from build123d import *

# Parameters (mm, degrees)
SKETCH_1_R      = 1
SKETCH_1_R_2    = 2
EXTRUDE_1_DEPTH = 2


with BuildPart() as part:
    # Эскиз1 → Бобышка-Вытянуть1 (new body)
    with BuildSketch(Plane(origin=(0, 0, 0), x_dir=(1, 0, 0), z_dir=(0, 1, 0))):
        with BuildLine():
            Line((8, 25.5), (48.3, 25.5))
            Line((48.3, 25.5), (48.3, 16))
            Line((48.3, 16), (56.3, 16))
            Line((56.3, 16), (56.3, 14))
            Line((56.3, 14), (48.3, 14))
            Line((48.3, 14), (48.3, 4.5))
            Line((48.3, 4.5), (8, 4.5))
            Line((8, 4.5), (8, 14))
            Line((8, 14), (0, 14))
            Line((0, 14), (0, 0))
            Line((0, 0), (75.8, 0))
            ThreePointArc((75.8, 0), (90.8, 15), (75.8, 30))
            Line((75.8, 30), (0, 30))
            Line((0, 30), (0, 16))
            Line((0, 16), (8, 16))
            Line((8, 16), (8, 25.5))
        make_face()
        with Locations(Location((3.4, 10, 0), (0, 0, 270))):
            Circle(SKETCH_1_R, mode=Mode.SUBTRACT)
        with Locations(Location((3.4, 20, 0), (0, 0, 270))):
            Circle(SKETCH_1_R, mode=Mode.SUBTRACT)
        with Locations(Location((52.6, 10, 0), (0, 0, 270))):
            Circle(SKETCH_1_R, mode=Mode.SUBTRACT)
        with Locations(Location((52.6, 20, 0), (0, 0, 270))):
            Circle(SKETCH_1_R, mode=Mode.SUBTRACT)
        with Locations(Location((75.8, 15, 0), (0, 0, 270))):
            Circle(SKETCH_1_R_2, mode=Mode.SUBTRACT)
    extrude(amount=EXTRUDE_1_DEPTH)


solid = part.part
CAD build for the part. Positions are in the model's coordinates, mm. A direction names the side the tool comes from. Round coordinates to 2 decimals unless told otherwise and drop trailing zeros. Loops run counter-clockwise (first coordinate to the right, second up) from the corner with the lowest first, then second, coordinate; pieces in that order, holes last. Notation, with made-up numbers: M -18,26.25 L 19,26.25 A29 ccw 19,55.25 Z; hole C 28.5,-18 d7. An arc over 180 degrees is marked long. One line per question, with ' | ' between items. Start each with the question number.
Item 1: Cut at A-A, the plane x = 39.5. Write the cut outline in (y, z).
Item 2: Cut at B-B, the plane y = 0.5. Write the cut outline in (x, z), plus the area to 3 significant figures.
Item 3: Wall check: line 1 (Z direction, x = 22, y = 0.35); line 2 (X direction, y = 1.55, z = -13.25); line 3 (X direction, y = 0.6, z = -10). Give the ranges that are in metal, low to high.
Item 4: Which spindle directions (+Z, -Z, +X, -X, +Y, -Y) get a long thin tool onto all of the face, cutting with end or side? Do faces 4 (the flat face through (48.3, 1, -9)), 5 (the cylindrical face through (90.796, 0.986, -14.67)), 6 (the flat face through (52, 1, -16)). Say none if no direction does.
Item 5: Cut at D-D, the plane z = -22.25. Write the cut outline in (x, y), plus the area to 3 significant figures.
Item 6: Cut at C-C, the plane x = 3.4. Write the cut outline in (y, z), plus the area to 3 significant figures.
Item 7: Two-plate mould, pull along X, no slides. Class faces 1 (the flat face through (38, 1, -30)), 2 (the cylindrical face through (2.8, 1, -10.8)), 3 (the flat face through (56.3, 1, -15)): pulls with the +X half, pulls with the -X half, needs draft (parallel to the pull), parting line crosses it, or undercut.
Item 8: Pin check, flat tips, straight feed: pin 1 Ø1 at (y, z) = (1.5, -18.5) entering from +X; pin 2 Ø0.6 at (y, z) = (1, -15) entering from -X; pin 3 Ø1 at (y, z) = (0.5, -9) entering from +X. Stop position of each tip, or through.
Responses:
1) outline: M 0,-30 L 2,-30 L 2,-25.5 L 0,-25.5 Z; M 0,-4.5 L 2,-4.5 L 2,0 L 0,0 Z
2) outline: M 0,-30 L 75.8,-30 A15 ccw 75.8,0 L 0,0 L 0,-14 L 8,-14 L 8,-4.5 L 48.3,-4.5 L 48.3,-14 L 56.3,-14 L 56.3,-16 L 48.3,-16 L 48.3,-25.5 L 8,-25.5 L 8,-16 L 0,-16 Z; hole C 3.4,-20 d2; hole C 3.4,-10 d2; hole C 52.6,-20 d2; hole C 52.6,-10 d2; hole C 75.8,-15 d4 | area: 1,720 mm²
3) line 1: z = -30 to -25.5, -4.5 to 0 | line 2: x = 0 to 8, 48.3 to 74.83, 76.77 to 90.7 | line 3: x = 0 to 2.4, 4.4 to 8, 48.3 to 51.6, 53.6 to 89.94
4) face 4: +Y, -Y | face 5: +X, +Y, -Y | face 6: -X, +Y, -Y
5) outline: M 0,0 L 8,0 L 8,2 L 0,2 Z; M 48.3,0 L 88.93,0 L 88.93,2 L 48.3,2 Z | area: 97.3 mm²
6) outline: M 0,-30 L 2,-30 L 2,-21 L 0,-21 Z; M 0,-19 L 2,-19 L 2,-16 L 0,-16 Z; M 0,-14 L 2,-14 L 2,-11 L 0,-11 Z; M 0,-9 L 2,-9 L 2,0 L 0,0 Z | area: 48.0 mm²
7) face 1: needs draft | face 2: undercut | face 3: pulls with the -X half
8) pin 1: stops at x = 90.5 | pin 2: stops at x = 56.3 | pin 3: stops at x = 89.76
